```python
from build123d import *

# Parameters (mm, degrees)
SKETCH_4_W      = 40.3
SKETCH_4_H      = 19.9
EXTRUDE_2_DEPTH = 37.5
EXTRUDE_START   = 27
SKETCH_5_W      = 54
SKETCH_5_H      = 19.9
SKETCH_5_R      = 2
EXTRUDE_3_DEPTH = 2.5
SKETCH_6_R      = 2.5
EXTRUDE_4_DEPTH = 5.5
EXTRUDE_START_2 = 2.37
SKETCH_8_R      = 2.25
EXTRUDE_5_DEPTH = 30.53
FILLET_1_R      = 2


with BuildPart() as part:
    # 草图4 → 凸台-拉伸2 (new body)
    with BuildSketch(Plane(origin=(0, 0, 0), x_dir=(1, 0, 0), z_dir=(0, 1, 0))):
        Rectangle(SKETCH_4_W, SKETCH_4_H)
    extrude(amount=EXTRUDE_2_DEPTH)

    # 草图5 → 凸台-拉伸3 (add)
    with BuildSketch(Plane(origin=(0, 0, 0), x_dir=(1, 0, 0), z_dir=(0, 1, 0)).offset(EXTRUDE_START)):
        Rectangle(SKETCH_5_W, SKETCH_5_H)
        with Locations(Location((24.3, 4.95, 0), (0, 0, 270))):
            Circle(SKETCH_5_R, mode=Mode.SUBTRACT)
        with Locations(Location((24.3, -4.95, 0), (0, 0, 90))):
            Circle(SKETCH_5_R, mode=Mode.SUBTRACT)
        with Locations(Location((-24.3, -4.95, 0), (0, 0, 270))):
            Circle(SKETCH_5_R, mode=Mode.SUBTRACT)
        with Locations(Location((-24.3, 4.95, 0), (0, 0, 90))):
            Circle(SKETCH_5_R, mode=Mode.SUBTRACT)
    extrude(amount=EXTRUDE_3_DEPTH)

    # 草图6 → 凸台-拉伸4 (add)
    with BuildSketch(Plane(origin=(0, 37.5, 0), x_dir=(1, 0, 0), z_dir=(0, 1, 0))):
        with Locations(Location((10, 0, 0), (0, 0, 90))):
            Circle(SKETCH_6_R)
    extrude(amount=EXTRUDE_4_DEPTH)

    # 草图8 → 凸台-拉伸5 (add)
    with BuildSketch(Plane(origin=(0, 32.9, 0), x_dir=(-1, 0, 0), z_dir=(0, -1, 0)).offset(EXTRUDE_START_2)):
        with Locations((-10, 0)):
            Circle(SKETCH_8_R)
    extrude(amount=EXTRUDE_5_DEPTH)

    # 圆角1
    fillet_1_edges = [part.edges().sort_by_distance(p)[0] for p in [
        (27, 28.25, -9.95),
        (-27, 28.25, 9.95),
        (27, 28.25, 9.95),
        (-27, 28.25, -9.95),
    ]]
    fillet(fillet_1_edges, radius=FILLET_1_R)


solid = part.part
```
The model under review builds one solid part; all positions refer to its coordinate system, in mm. A direction names the side the tool comes from. Round coordinates to 2 decimals unless told otherwise and drop trailing zeros. Loops run counter-clockwise (first coordinate to the right, second up) from the corner with the lowest first, then second, coordinate; pieces in that order, holes last. Notation, with made-up numbers: M 4,81.5 L 26,81.5 A18 ccw 26,102.5 Z; hole C 50.25,12 d5. An arc over 180 degrees is marked long. Put each result on its own line as item: value.
Q1. Mouldability with a two-part tool opening along X and no side actions: class faces 4 (the flat face through (-20.15, 13, 0)), 5 (the cylindrical face through (26.252, 28.232, 5.384)), 6 (the flat face through (0, 18, 9.95)) as released by +X, released by -X, zero draft, split by the parting line, or undercut.
Result set:
face 4: released by -X
face 5: undercut
face 6: zero draft
Q2. To check wall thickness, follow L1, parallel to X at y = 28.55, z = -4.95; L2, parallel to Y at x = -17, z = 0.75; L3, parallel to Y at x = 24, z = -1.75. State the ranges of each line that lie inside material, in increasing order.
Result set:
L1: x = -27 to -26.3, -22.3 to 22.3, 26.3 to 27
L2: y = 0 to 37.5
L3: y = 27 to 29.5
Q3. Machinability: for faces 1 (the flat face through (-24, 27, 0)), 2 (the flat face through (24, 27, 0)), 3 (the flat face through (24, 29.5, 0)), which of the approach directions +Z, -Z, +X, -X, +Y, -Y give a long, thin tool a straight path to every point of the face, cutting with its end or side? Answer none if there is none.
Result set:
face 1: +Z, -Z, -X, -Y
face 2: +Z, -Z, +X, -Y
face 3: +Z, -Z, +X, +Y
Q4. Consider section A-A, the plane x = 24.3. Give the boundary of the cut face in (y, z).
Result set:
outline: M 27,-9.95 L 29.5,-9.95 L 29.5,-6.95 L 27,-6.95 Z; M 27,-2.95 L 29.5,-2.95 L 29.5,2.95 L 27,2.95 Z; M 27,6.95 L 29.5,6.95 L 29.5,9.95 L 27,9.95 Z
Q5. For pin 1 (7.5 mm diameter, centred on x = 23.5, z = 4, fed in from +Y); pin 2 (4 mm diameter, centred on y = 34.5, z = 5, fed in from +X); pin 3 (2.5 mm diameter, centred on y = 31.5, z = 0.5, fed in from -X), all flat-tipped, find the tip position at first contact; note any pin that passes through.
Result set:
pin 1: stops at y = 37.5
pin 2: stops at x = 20.15
pin 3: stops at x = -20.15
Q6. Consider section B-B, the plane z = -4.95. Give the boundary of the cut face in (x, y), then the cut area to 3 significant figures.
Result set:
outline: M -27,27 L -26.3,27 L -26.3,29.5 L -27,29.5 Z; M -22.3,27 L -20.15,27 L -20.15,0 L 20.15,0 L 20.15,27 L 22.3,27 L 22.3,29.5 L 20.15,29.5 L 20.15,37.5 L -20.15,37.5 L -20.15,29.5 L -22.3,29.5 Z; M 26.3,27 L 27,27 L 27,29.5 L 26.3,29.5 Z
area: 1,530 mm²
Q7. Consider section D-D, the plane x = 10. Give the boundary of the cut face in (y, z), then the cut area to 3 significant figures.
Result set:
outline: M 0,-9.95 L 37.5,-9.95 L 37.5,-2.5 L 43,-2.5 L 43,2.5 L 37.5,2.5 L 37.5,9.95 L 0,9.95 Z
area: 774 mm²
Q8. Consider section C-C, the plane z = 0. Give the boundary of the cut face in (x, y).
Result set:
outline: M -27,27 L -20.15,27 L -20.15,0 L 20.15,0 L 20.15,27 L 27,27 L 27,29.5 L 20.15,29.5 L 20.15,37.5 L 12.5,37.5 L 12.5,43 L 7.5,43 L 7.5,37.5 L -20.15,37.5 L -20.15,29.5 L -27,29.5 Z
